Verification items for the finished model (mm, model axes). Face numbers are marked on the shaded views. A direction names the side the tool comes from. Coordinates: 2 decimals unless noted, no trailing zeros. Write each loop counter-clockwise with the first axis right and the second up, starting at its lowest first coordinate (ties: lowest second). Pieces come first, ordered by that corner, then holes. Notation, with made-up numbers: (57, -38.5) - (64, -38.5) arc R10 ccw to (64, -19.5) - close; hole circle Ø1 at (-1, -40). An arc over 180 degrees is marked (long way). Answer as CSV lines item,"result". Start each with the question number.
Autodesk Inventor part; units mm, degrees
ref_plane "YZ Plane" through (0, 0, 0) normal (1, 0, 0) x (0, 1, 0)
ref_plane "XZ Plane" through (0, 0, 0) normal (0, 1, 0) x (-1, 0, 0)
sketch "Skizze1" plane through (0, 0, 0) normal (0, 0, 1) x (1, 0, 0)
  line L0 (0, 0) -> (0, 22)
  line L1 (0, 22) -> (107, 22)
  line L2 (107, 22) -> (107, 30)
  line L3 (107, 30) -> (131.65, 30)
  line L4 (131.65, 30) -> (131.65, 36.5)
  line L5 (131.65, 36.5) -> (153.65, 36.5)
  line L6 (153.65, 36.5) -> (153.65, 30)
  line L7 (153.65, 30) -> (178.3, 30)
  line L8 (178.3, 30) -> (178.3, 0)
  line L9 (178.3, 0) -> (0, 0)
  line L10 (-35.66, 0) -> (213.96, 0)
revolve "Umdrehung1" add sketch "Skizze1" angle 360 about axis through (-10, 0, 0) along (1, 0, 0)
ref_plane "Arbeitsebene1" through (0, 0, 22) normal (0, 0, 1) x (1, 0, 0)
sketch "Skizze2" plane through (0, 0, 22) normal (0, 0, 1) x (1, 0, 0)
  line L0 (8.5, 0) -> (98.5, 0) construction
  line L1 (14.5, -6) -> (92.5, -6)
  line L2 (92.5, 6) -> (14.5, 6)
  arc A0 (14.5, 6) -> (14.5, -6) centre (14.5, 0) ccw
  arc A1 (92.5, -6) -> (92.5, 6) centre (92.5, 0) ccw
  point P0 (53.5, 0)
extrude "Extrusion1" cut sketch "Skizze2" against normal blind 5
properties part number "shaft_6"
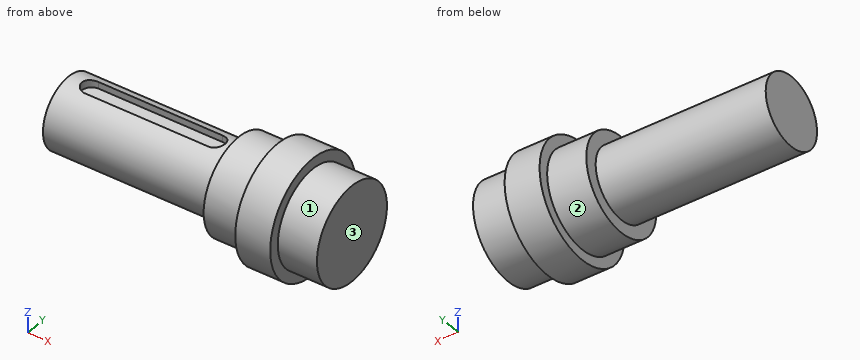
1. Scan lines: line 1 along X through (y, z) = (-3, 24); line 2 along Y through (x, z) = (147, 6); line 3 along Y through (x, z) = (27.5, -10). Record each from-to range of solid material in increasing order. Write a range as from..to.
2. Access from +Z, -Z, +X, -X, +Y, -Y to the whole of each face (thin tool, end or side, straight path). Record for the marked faces 1, 2 and 3.
3. Cross-section at A-A (y = 0). Record the cut outline in (x, z).
4. Cross-section at D-D (x = 24). Record the cut outline in (y, z).
5. Cross-section at C-C (z = -24). Record the cut outline in (x, y).
6. Depth check by flat-ended pin: P1, Ø3.5, axis at x = 34.5, y = 1.5, coming from the +Z side; P2, Ø12, axis at x = 52.5, z = 22, coming from the -Y side; P3, Ø3.5, axis at x = 65, z = 18, coming from the -Y side. Enter the tip coordinate at first touch or a pass-through.
7. Cross-section at B-B (z = 0). Record the cut outline in (x, y), and give its area (3 significant figures).
Completed:
1,line 1,"x = 107..178.3"
1,line 2,"y = -36..36"
1,line 3,"y = -19.6..19.6"
2,face 1,"+X"
2,face 2,"-X"
2,face 3,"+Z, -Z, +X, +Y, -Y"
3,outline,"(0, -22) - (107, -22) - (107, -30) - (131.65, -30) - (131.65, -36.5) - (153.65, -36.5) - (153.65, -30) - (178.3, -30) - (178.3, 30) - (153.65, 30) - (153.65, 36.5) - (131.65, 36.5) - (131.65, 30) - (107, 30) - (107, 22) - (98.5, 22) - (98.5, 17) - (8.5, 17) - (8.5, 22) - (0, 22) - close"
4,outline,"(-6, 17) - (-6, 21.17) arc R22 ccw (long way) to (6, 21.17) - (6, 17) - close"
5,outline,"(107, -18) - (131.65, -18) - (131.65, -27.5) - (153.65, -27.5) - (153.65, -18) - (178.3, -18) - (178.3, 18) - (153.65, 18) - (153.65, 27.5) - (131.65, 27.5) - (131.65, 18) - (107, 18) - close"
6,P1,"stops at z = 17"
6,P2,"stops at y = -15.1"
6,P3,"stops at y = -14.83"
7,outline,"(0, -22) - (107, -22) - (107, -30) - (131.65, -30) - (131.65, -36.5) - (153.65, -36.5) - (153.65, -30) - (178.3, -30) - (178.3, 30) - (153.65, 30) - (153.65, 36.5) - (131.65, 36.5) - (131.65, 30) - (107, 30) - (107, 22) - (0, 22) - close"
7,area,"9,270 mm2"
